```python
from build123d import *

# Parameters (mm, degrees)
ESTRUSIONE_ESTRUSIONE1_DEPTH = 120
TAGLIO_ESTRUSIONE2_REACH     = 166.924
SCHIZZO6_R                   = 7.75
TAGLIO_ESTRUSIONE3_REACH     = 166.924
SCHIZZO7_R                   = 9.5
FORO_PER_VITE_M4_2_D         = 4.5
SCHIZZO12_R                  = 3
TAGLIO_ESTRUSIONE4_DEPTH     = 10
SCHIZZO14_R                  = 2.6
TAGLIO_ESTRUSIONE5_DEPTH     = 10
SMUSSO2_SIZE                 = 1
FORO_FILETTATO_M3_1_D        = 2.5
FORO_FILETTATO_M3_1_DEPTH    = 10
FORO_FILETTATO_M3_1_TIP      = 0.751075774


with BuildPart() as part:
    # Schizzo1 → Estrusione-Estrusione1 (new body)
    with BuildSketch(Plane.XY):
        Polygon((0, 0), (-80, 0), (-80, -8), (-8, -8), (-8, -80), (0, -80), align=None)
    extrude(amount=ESTRUSIONE_ESTRUSIONE1_DEPTH)

    # Schizzo6 → Taglio-Estrusione2 (cut, up to next)
    with BuildSketch(Plane(origin=(0, 0, 0), x_dir=(1, 0, 0), z_dir=(0, 1, 0)), mode=Mode.PRIVATE) as taglio_estrusione2_sk1:
        with Locations(Location((-23, -21, 0), (0, 0, 180))):
            Circle(SCHIZZO6_R)
    taglio_estrusione2_tool1 = extrude(taglio_estrusione2_sk1.sketch, amount=-TAGLIO_ESTRUSIONE2_REACH, mode=Mode.PRIVATE) & part.part
    # Schizzo6 → Taglio-Estrusione2 (cut, up to next)
    with BuildSketch(Plane(origin=(0, 0, 0), x_dir=(1, 0, 0), z_dir=(0, 1, 0)), mode=Mode.PRIVATE) as taglio_estrusione2_sk2:
        with Locations(Location((-23, -99, 0), (0, 0, 180))):
            Circle(SCHIZZO6_R)
    taglio_estrusione2_tool2 = extrude(taglio_estrusione2_sk2.sketch, amount=-TAGLIO_ESTRUSIONE2_REACH, mode=Mode.PRIVATE) & part.part
    add(taglio_estrusione2_tool1.solids().sort_by_distance((-23, 0, 21))[0], mode=Mode.SUBTRACT)
    add(taglio_estrusione2_tool2.solids().sort_by_distance((-23, 0, 99))[0], mode=Mode.SUBTRACT)

    # Schizzo7 → Taglio-Estrusione3 (cut, up to next)
    with BuildSketch(Plane(origin=(0, 0, 0), x_dir=(1, 0, 0), z_dir=(0, 1, 0)), mode=Mode.PRIVATE) as taglio_estrusione3_sk1:
        with Locations(Location((-29, -60, 0), (0, 0, 180))):
            Circle(SCHIZZO7_R)
    taglio_estrusione3_tool1 = extrude(taglio_estrusione3_sk1.sketch, amount=-TAGLIO_ESTRUSIONE3_REACH, mode=Mode.PRIVATE) & part.part
    add(taglio_estrusione3_tool1.solids().sort_by_distance((-29, 0, 60))[0], mode=Mode.SUBTRACT)

    # Foro per Vite M4-2 (through all)
    with Locations(Plane(origin=(0, 0, 0), x_dir=(1, 0, 0), z_dir=(0, 1, 0))):
        with Locations((-29, -47), (-42, -60), (-29, -73), (-16, -60), (-29, -60)):
            Hole(FORO_PER_VITE_M4_2_D / 2)

    # Schizzo12 → Taglio-Estrusione4 (cut)
    with BuildSketch(Plane(origin=(0, 0, 0), x_dir=(0, 0, -1), z_dir=(1, 0, 0))):
        with Locations((-113.75, -19)):
            Circle(SCHIZZO12_R)
        with Locations(Location((-83.25, -19, 0), (0, 0, 90))):
            Circle(SCHIZZO12_R)
        with Locations((-36.75, -19)):
            Circle(SCHIZZO12_R)
        with Locations(Location((-6.25, -19, 0), (0, 0, 90))):
            Circle(SCHIZZO12_R)
        with Locations((-83.25, -69)):
            Circle(SCHIZZO12_R)
        with Locations(Location((-113.75, -69, 0), (0, 0, 90))):
            Circle(SCHIZZO12_R)
        with Locations((-6.25, -69)):
            Circle(SCHIZZO12_R)
        with Locations(Location((-36.75, -69, 0), (0, 0, 90))):
            Circle(SCHIZZO12_R)
    extrude(amount=-TAGLIO_ESTRUSIONE4_DEPTH, mode=Mode.SUBTRACT)

    # Schizzo14 → Taglio-Estrusione5 (cut)
    with BuildSketch(Plane(origin=(0, 0, 0), x_dir=(1, 0, 0), z_dir=(0, 1, 0))):
        with Locations(Location((-70, -18, 0), (0, 0, 180))):
            Circle(SCHIZZO14_R)
        with Locations(Location((-70, -60, 0), (0, 0, 180))):
            Circle(SCHIZZO14_R)
        with Locations(Location((-70, -102, 0), (0, 0, 180))):
            Circle(SCHIZZO14_R)
        with Locations(Location((-55, -35, 0), (0, 0, 180))):
            Circle(SCHIZZO14_R)
        with Locations(Location((-55, -85, 0), (0, 0, 180))):
            Circle(SCHIZZO14_R)
    extrude(amount=-TAGLIO_ESTRUSIONE5_DEPTH, mode=Mode.SUBTRACT)

    # Smusso2
    smusso2_edges = [part.edges().sort_by_distance(p)[0] for p in [
        (-19.5, 0, 60),
    ]]
    chamfer(smusso2_edges, length=SMUSSO2_SIZE)

    # Foro filettato M3-1
    with Locations(Plane.XY.offset(120)):
        with Locations((-10, -4), (-29, -4)):
            Hole(FORO_FILETTATO_M3_1_D / 2, depth=FORO_FILETTATO_M3_1_DEPTH)
            with Locations((0, 0, -(FORO_FILETTATO_M3_1_DEPTH + FORO_FILETTATO_M3_1_TIP / 2))):  # 118° drill point
                Cone(0, FORO_FILETTATO_M3_1_D / 2, FORO_FILETTATO_M3_1_TIP, mode=Mode.SUBTRACT)


solid = part.part
```
Read the model definition and answer for the solid it produces. Units are mm, in the model's axes. A direction names the side the tool comes from. Give positions to 0.01 mm unless a question says otherwise; leave off trailing zeros. Loops run counter-clockwise (first coordinate to the right, second up) from the corner with the lowest first, then second, coordinate; pieces in that order, holes last.
Item 1: The part is cut by section D-D (y = -51). Write down the section's boundary in (x, z).
Item 2: Find the intervals of material crossed by line 1 along Y through (x, z) = (-3, 83); line 2 along X through (y, z) = (-4, 116.5); line 3 along Z through (x, y) = (-42, -4), in increasing order.
Item 3: Each of these flat-tipped pins is pushed along its axis until it touches: pin 1 Ø3 at (x, y) = (-29, -4) entering from -Z; pin 2 Ø4.5 at (x, z) = (-55, 35) entering from -Y; pin 3 Ø25 at (x, z) = (-23, 99) entering from -Y. Where does it stop, or does it pass through?
Item 4: The part is cut by section C-C (z = 47). Write down the section's boundary in (x, y), and give its area (3 significant figures).
Item 5: The part is cut by section B-B (z = 6.25). Write down the section's boundary in (x, y).
Item 6: The mould has two halves that part along Z. Classify faces 1 (the flat face through (-4, -80, 59)), 2 (the flat face through (-25, -7, 120)), 3 (the cylindrical face through (-3.94, -71.21, 115.78)): released by +Z, released by -Z, zero draft, split by the parting line, or undercut.
Item 7: The part is cut by section A-A (z = 113.75). Write down the section's boundary in (x, y), and give its area (3 significant figures).
Item 8: For faces 4 (the cylindrical face through (-3.944, -18.868, 39.747)), 5 (the cylindrical face through (-30.155, -4.479, 114.93)), 6 (the flat face through (-8, -43, 59)), determine the directions among +Z, -Z, +X, -X, +Y, -Y from which every point of the face is accessible in a straight line to the end or side of a thin tool.
Taken from the geometry:
1. outline: (-8, 0) - (0, 0) - (0, 120) - (-8, 120) - close
2. line 1: y = -80 to -71.99, -66.01 to -21.99, -16.01 to 0
2. line 2: x = -80 to -30.25, -27.75 to -11.25, -8.75 to 0
2. line 3: z = 0 to 57.75, 62.25 to 120
3. pin 1: stops at z = 0
3. pin 2: passes through
3. pin 3: stops at y = -8
4. outline: (-80, -8) - (-31.25, -8) - (-31.25, 0) - (-80, 0) - close; (-26.75, -8) - (-8, -8) - (-8, -80) - (0, -80) - (0, 0) - (-26.75, 0) - close
4. area: 1,180 mm2
5. outline: (-80, -8) - (-8, -8) - (-8, -16) - (0, -16) - (0, 0) - (-80, 0) - close; (-8, -80) - (0, -80) - (0, -72) - (-8, -72) - close; (-8, -66) - (0, -66) - (0, -22) - (-8, -22) - close
6. face 1: zero draft
6. face 2: released by +Z
6. face 3: undercut
7. outline: (-80, -8) - (-8, -8) - (-8, -16) - (0, -16) - (0, 0) - (-80, 0) - close; (-8, -80) - (0, -80) - (0, -72) - (-8, -72) - close; (-8, -66) - (0, -66) - (0, -22) - (-8, -22) - close; hole circle Ø2.5 at (-29, -4); hole circle Ø2.5 at (-10, -4)
7. area: 1,110 mm2
8. face 4: +X, -X
8. face 5: +Z
8. face 6: +Z, -Z, -X, -Y
